Input: dimensioned drawing with shaded views. Units: mm. Origin: part minimum x, y, z. A direction names the side the tool comes from. Coordinates: 2 decimals unless noted, no trailing zeros. Loops run counter-clockwise (first coordinate to the right, second up) from the corner with the lowest first, then second, coordinate; pieces in that order, holes last.
Item 1: Section query B-B, the plane x = 11.5. Return the cut outline in (y, z).
Item 2: Section query C-C, the plane y = 47. Return the cut outline in (x, z).
Item 3: Pull-direction query (Y, two-part tool) for the marked faces 3, 4 and 5; classes: +Y half, -Y half, draft (parallel to the pull), parting line (faces both ways), or undercut.
Item 4: Line query: probe 1 along X at (y, z) = (12, 4); probe 2 along Y at (x, z) = (2.5, 8.75); probe 3 along Y at (x, z) = (22.25, 3.5). Output: solid intervals per line, ascending.
Item 5: Pin query (flat end, axial travel): pin 1 Ø0.5 at (x, z) = (18, 8.5) entering from +Y; pin 2 Ø2 at (x, y) = (9, 15.5) entering from +Z. Return the tip coordinate at first contact, or that it passes through.
Item 6: Section query D-D, the plane z = 8.25. Return the cut outline in (x, y).
Item 7: Reachability of the marked faces 1 and 2 from +Z, -Z, +X, -X, +Y, -Y: full face, straight path, thin tool, end or side. Return the list, or none.
Item 8: Section query A-A, the plane z = 4.5. Return the cut outline in (x, y).
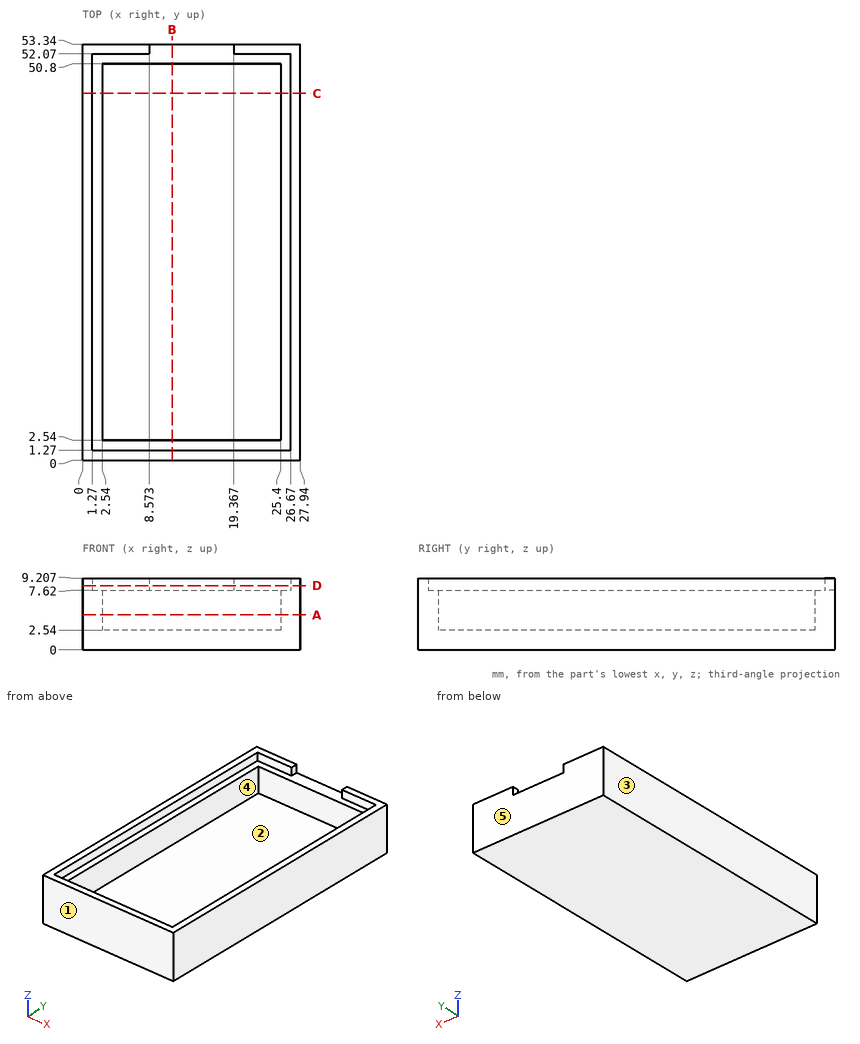
Verdict:
1. outline: (0, 0) - (53.34, 0) - (53.34, 7.62) - (50.8, 7.62) - (50.8, 2.54) - (2.54, 2.54) - (2.54, 7.62) - (1.27, 7.62) - (1.27, 9.21) - (0, 9.21) - close
2. outline: (0, 0) - (27.94, 0) - (27.94, 9.21) - (26.67, 9.21) - (26.67, 7.62) - (25.4, 7.62) - (25.4, 2.54) - (2.54, 2.54) - (2.54, 7.62) - (1.27, 7.62) - (1.27, 9.21) - (0, 9.21) - close
3. face 3: draft
3. face 4: undercut
3. face 5: +Y half
4. probe 1: x = 0 to 2.54, 25.4 to 27.94
4. probe 2: y = 0 to 1.27, 52.07 to 53.34
4. probe 3: y = 0 to 2.54, 50.8 to 53.34
5. pin 1: stops at y = 1.27
5. pin 2: stops at z = 2.54
6. outline: (0, 0) - (27.94, 0) - (27.94, 53.34) - (19.37, 53.34) - (19.37, 52.07) - (26.67, 52.07) - (26.67, 1.27) - (1.27, 1.27) - (1.27, 52.07) - (8.57, 52.07) - (8.57, 53.34) - (0, 53.34) - close
7. face 1: +Z, -Z, +X, -X, -Y
7. face 2: +Z
8. outline: (0, 0) - (27.94, 0) - (27.94, 53.34) - (0, 53.34) - close; hole (2.54, 2.54) - (25.4, 2.54) - (25.4, 50.8) - (2.54, 50.8) - close
